from build123d import *

# Parameters (mm, degrees)
F1_DEPTH       = 100
F3_D           = 13
F3_DEPTH       = 10
F3_CSINK_D     = 18
F3_CSINK_ANGLE = 90
F4_SIZE        = 0.5
F5_R           = 0.25


with BuildPart() as f1:
    # F0 (on Front) → F1 (new body)
    with BuildSketch(Plane.XZ):
        Polygon((0, 50), (0, 0), (35, 0), (35, 4.5), (6, 4.5), (6, 50), align=None)
    extrude(amount=F1_DEPTH)

    # F3
    with Locations(Plane.YZ.offset(6)):
        with Locations((-87.5, 28.514809), (-12.5, 27.276697)):
            CounterSinkHole(F3_D / 2, F3_CSINK_D / 2, depth=F3_DEPTH, counter_sink_angle=F3_CSINK_ANGLE)

    # F4
    f4_edges = [f1.edges().sort_by_distance(p)[0] for p in [
        (20.5, -100, 4.5),
        (35, -50, 4.5),
        (20.5, 0, 4.5),
    ]]
    chamfer(f4_edges, length=F4_SIZE)

    # F5
    f5_edges = [f1.edges().sort_by_distance(p)[0] for p in [
        (3, -100, 50),
        (3, 0, 50),
        (35, -100, 2),
        (35, 0, 2),
    ]]
    fillet(f5_edges, radius=F5_R)


solid = f1.part
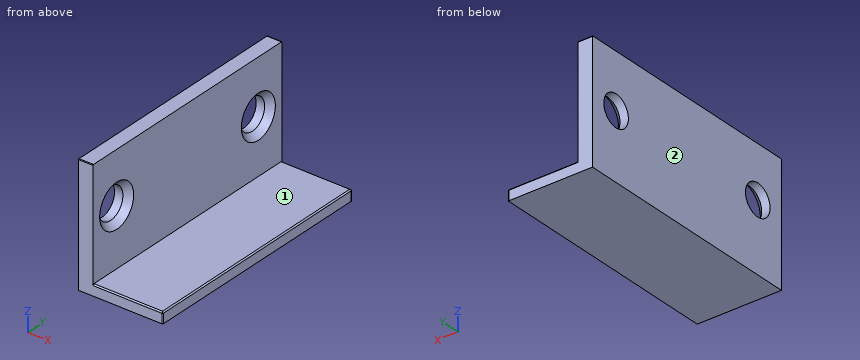
Input: part model. Units: mm. Frame: model coordinates. Face numbers are marked on the shaded views. A direction names the side the tool comes from. Give positions to 0.01 mm unless a question says otherwise; leave off trailing zeros. Order: outer loops, then holes, each group sorted by start corner. A loop starts at its lowest first (then second) coordinate and runs counter-clockwise, first axis right, second up. Notation, with made-up numbers: (43.5, 64.5) - (87.5, 64.5) arc R18 cw to (87.5, 70.5) - close; hole circle Ø7 at (87, 33). An arc over 180 degrees is marked (long way). Answer as a JSON object with one key per item and string values. Group by question number.
Q1. Set-up query: the marked faces 1 and 2. Return all of +Z, -Z, +X, -X, +Y, -Y with unobstructed straight access to the full face (end or side cutting, diameter ignored); none if empty.
Q2. Cut plane D-D, the plane z = 9. Output: boundary loops of the cut face in (x, y).
Q3. Cut plane A-A, the plane y = -87.5. Output: boundary loops of the cut face in (x, z), then the cut area to 3 significant figures.
Q4. Cut plane B-B, the plane y = -60.5. Output: boundary loops of the cut face in (x, z).
Q5. First-contact query: pin 1 Ø12 at (x, z) = (16.5, 37) entering from -Y; pin 2 Ø3 at (y, z) = (-55.5, 8) entering from +X; pin 3 Ø8.5 at (x, y) = (27, -54) entering from +Z. Flat tips, straight axial feed; report the tip coordinate or a pass-through.
Q6. Line query: probe 1 along Z at (x, y) = (0.9, -87.5); probe 2 along Z at (x, y) = (1, -12); probe 3 along Z at (x, y) = (25, -87). Output: solid intervals per line, ascending.
Q7. Cut plane C-C, the plane x = 13.5. Output: boundary loops of the cut face in (y, z), then the cut area to 3 significant figures.
Results:
{
 "1": {"face 1": "+Z, +X, +Y, -Y", "face 2": "+Z, -Z, -X, +Y, -Y"},
 "2": {"outline": "(0, -100) - (6, -100) - (6, 0) - (0, 0) - close"},
 "3": {"outline": "(0, 0) - (35, 0) - (35, 4) - (34.5, 4.5) - (6, 4.5) - (6, 19.51) - (3.5, 22.01) - (0, 22.01) - close; (0, 35.01) - (3.5, 35.01) - (6, 37.51) - (6, 50) - (0, 50) - close", "area": "346 mm^2"},
 "4": {"outline": "(0, 0) - (35, 0) - (35, 4) - (34.5, 4.5) - (6, 4.5) - (6, 50) - (0, 50) - close"},
 "5": {"pin 1": "through", "pin 2": "x = 6", "pin 3": "z = 4.5"},
 "6": {"probe 1": "0 to 22.01, 35.01 to 50", "probe 2": "0 to 20.8, 33.76 to 50", "probe 3": "0 to 4.5"},
 "7": {"outline": "(-100, 0) - (0, 0) - (0, 4) - (-0.5, 4.5) - (-99.5, 4.5) - (-100, 4) - close", "area": "450 mm^2"}
}
